```python
from build123d import *

# Parameters (mm, degrees)
SKETCH1_R           = 29
SKETCH1_R_2         = 28
EXTRUDE_THIN1_DEPTH = 10
SKETCH16_R          = 1.5
CUT_EXTRUDE2_DEPTH  = 26.001091713
SKETCH6_R           = 1.5
CUT_EXTRUDE1_DEPTH  = 1


with BuildPart() as part:
    # Sketch1 → Extrude-Thin1 (new body, symmetric)
    with BuildSketch(Plane.XY):
        Circle(SKETCH1_R)
        Circle(SKETCH1_R_2, mode=Mode.SUBTRACT)
    extrude(amount=EXTRUDE_THIN1_DEPTH, both=True)

    # Sketch5 → Revolve-Thin4 (revolve)
    with BuildSketch(Plane(origin=(0, 0, 0), x_dir=(0, 0, -1), z_dir=(1, 0, 0))):
        with BuildLine():
            Line((10, 29), (10, 0))
            Line((10, 0), (25, 0))
            ThreePointArc((25, 0), (21.088709123, 16.356228857), (10, 29))
        make_face()
        with BuildLine():
            Line((11, 27.016767879), (11, 1))
            Line((11, 1), (23.993391354, 1))
            ThreePointArc((23.993391354, 1), (20.418624313, 15.467664449), (11, 27.016767879))
        make_face(mode=Mode.SUBTRACT)
    revolve(axis=Axis((0, 0, 0), (0, 0, -1)))

    # Sketch7 → Cut-Revolve1 (revolve, cut)
    with BuildSketch(Plane(origin=(0, 0, 0), x_dir=(0, 0, -1), z_dir=(1, 0, 0))):
        with BuildLine():
            Line((10, 0), (24, 0))
            ThreePointArc((24, 0), (20.411655154, 15.485438383), (10, 27.496785417))
            Line((10, 27.496785417), (10, 0))
        make_face()
    revolve(axis=Axis((0, 0, -10), (0, 0, -1)), mode=Mode.SUBTRACT)

    # Sketch16 → Cut-Extrude2 (cut, through all)
    with BuildSketch(Plane.XY):
        Circle(SKETCH16_R)
    extrude(amount=-CUT_EXTRUDE2_DEPTH, mode=Mode.SUBTRACT)

    # Sketch6 → Cut-Extrude1 (cut)
    with BuildSketch(Plane.XY.offset(-10)):
        Circle(SKETCH6_R)
    extrude(amount=-CUT_EXTRUDE1_DEPTH, mode=Mode.SUBTRACT)


solid = part.part
```
Input: part model. Units: mm. Frame: model coordinates. A direction names the side the tool comes from. Round coordinates to 2 decimals unless told otherwise and drop trailing zeros. Loops run counter-clockwise (first coordinate to the right, second up) from the corner with the lowest first, then second, coordinate; pieces in that order, holes last. Notation, with made-up numbers: (0, 6.25) -> (32, 6.25) arc R27 ccw to (32, 31.25) -> close; hole circle Ø8 at (30.25, -39). An arc over 180 degrees is marked (long way). Write each question's results on one line, items separated by ' | '.
1. Ray query, line 1 (Y direction, x = 0, z = -2.5); line 2 (Y direction, x = 13, z = 8). Return the intervals inside material, ascending. Write a range as from..to.
Geometry results:
line 1: -29..-28, 28..29 | line 2: -25.92..-24.8, 24.8..25.92
2. Mould query, pull axis X, two halves, no side actions, for faces 1 (the face through (25.865, -10.724, -0.14)), 2 (the face through (-15, 24, 10)), 3 (the face through (13.38, -25.73, 0.14)). Classes: +X half, -X half, draft (parallel to the pull), parting line (faces both ways), or undercut.
Geometry results:
face 1: undercut | face 2: draft | face 3: parting line
3. Section A-A (z = 8). Return loops of the section in (x, y).
Geometry results:
outline: circle Ø58 at (0, 0); hole circle Ø56 at (0, 0)
4. Set-up query: faces 4 (the face through (-20.6, 18.5, -10)), 5 (the face through (-1.5, 0.07, -24.48)). Return all of +Z, -Z, +X, -X, +Y, -Y with unobstructed straight access to the full face (end or side cutting, diameter ignored); none if empty.
Geometry results:
face 4: +Z | face 5: +Z, -Z
5. First-contact query: P1, Ø5, axis at x = 23, y = -15, coming from the -Z side; P2, Ø5, axis at x = 7.5, z = -5.5, coming from the +Y side; P3, Ø5, axis at x = 0, y = 0, coming from the -Z side; P4, Ø10, axis at x = -6.5, z = -20.5, coming from the -Y side. Flat tips, straight axial feed; report the tip coordinate or a pass-through.
Geometry results:
P1: z = -14.82 | P2: y = 28.57 | P3: z = -24.98 | P4: y = -23.51
